Can you work these out from the model? Positions are in its coordinate system, mm. A direction names the side the tool comes from. Coordinates: 2 decimals unless noted, no trailing zeros. Order: outer loops, then holes, each group sorted by start corner. A loop starts at its lowest first (then second) coordinate and runs counter-clockwise, first axis right, second up. Notation, with made-up numbers: (-9.5, 14) -> (-4.5, 14) arc R26 cw to (-4.5, 46) -> close; hole circle Ø5 at (-32.75, 27.5). An arc over 180 degrees is marked (long way). Write item = value, one per line.
```python
from build123d import *

# Parameters (mm, degrees)
F0_W     = 7.62
F0_H     = 12.7
F1_DEPTH = 5.08
F2_W     = 5.08
F2_H     = 2.54
F3_DEPTH = 25.4
F5_DEPTH = 2.54


# Not quite as in the source:
# - a feature names something its author has since deleted; it is built from what else it names


with BuildPart() as f1:
    # F0 (on Top) → F1 (new body)
    with BuildSketch(Plane.XY):
        with Locations((-65.9446567297, 13.238232059)):
            Rectangle(F0_W, F0_H)
    extrude(amount=F1_DEPTH)

    # F2 (on face) → F3 (join)
    with BuildSketch(Plane(origin=(-69.7546567297, 0, 0), x_dir=(0, -1, 0), z_dir=(-1, 0, 0))):
        with Locations((-13.238232059, 1.27)):
            Rectangle(F2_W, F2_H)
    extrude(amount=F3_DEPTH)

    # F4 (on face) → F5 (join)
    with BuildSketch(Plane(origin=(0, 0, 0), x_dir=(1, 0, 0), z_dir=(0, 0, -1))):
        with BuildLine():
            Line((-93.5208049366, -15.778232059), (-95.1546567297, -15.778232059))
            Line((-95.1546567297, -15.778232059), (-95.1546567297, -10.698232059))
            ThreePointArc((-95.1546567297, -10.698232059), (-100.7342725481, -24.1686162406), (-114.2046567297, -29.748232059))
            Line((-114.2046567297, -29.748232059), (-114.2046567297, -31.9967795447))
            ThreePointArc((-114.2046567297, -31.9967795447), (-101.0625202258, -27.4586727786), (-93.5208049366, -15.778232059))
        make_face()
    extrude(amount=-F5_DEPTH)


solid = f1.part
```
Item 1: If we mould it in two halves opening along X, with no side actions, what happens to faces 1 (the flat face through (-66, 6.888, 3)), 2 (the flat face through (-81, 15.778, 1)), 3 (the flat face through (-62.135, 13, 3))? For each: pulls with the +X half, pulls with the -X half, needs draft (parallel to the pull), parting line crosses it, or undercut.
A:
face_1 = needs draft
face_2 = undercut
face_3 = pulls with the +X half
Item 2: I want a section at D-D, the plane z = 3.4. Please give me the cut outline in (x, y), plus the area to 3 significant figures.
A:
outline = (-69.75, 6.89) -> (-62.13, 6.89) -> (-62.13, 19.59) -> (-69.75, 19.59) -> close
area = 96.8 mm2
Item 3: I want a section at B-B, the plane y = 17.25. Please give me the cut outline in (x, z), plus the area to 3 significant figures.
A:
outline = (-96.32, 0) -> (-93.94, 0) -> (-93.94, 2.54) -> (-96.32, 2.54) -> close; (-69.75, 0) -> (-62.13, 0) -> (-62.13, 5.08) -> (-69.75, 5.08) -> close
area = 44.7 mm2
Item 4: I want a section at A-A, the plane z = 0.65. Please give me the cut outline in (x, y), plus the area to 3 significant figures.
A:
outline = (-114.2, 29.75) arc R19.05 cw to (-95.15, 10.7) -> (-69.75, 10.7) -> (-69.75, 6.89) -> (-62.13, 6.89) -> (-62.13, 19.59) -> (-69.75, 19.59) -> (-69.75, 15.78) -> (-93.52, 15.78) arc R21.3 ccw to (-114.2, 32) -> close
area = 287 mm2
Item 5: If I drill on probe 1 along X at (y, z) = (16, 1.85); probe 2 along X at (y, z) = (16.25, 1.7); probe 3 along Y at (x, z) = (-73, 0.6), over which ranges is the centre line in solid material (lowest first)?
A:
probe_1 = -95.91 to -93.58, -69.75 to -62.13
probe_2 = -95.98 to -93.64, -69.75 to -62.13
probe_3 = 10.7 to 15.78
Item 6: I'm going to push flat-ended pins straight in: P1, Ø1.5, axis at x = -66, z = 3, coming from the +Y side; P2, Ø1.3, axis at x = -77, z = 1, coming from the -Y side; P3, Ø1, axis at x = -99.5, z = 2.5, coming from the +Y side; P4, Ø1.5, axis at y = 29, z = 4.5, coming from the -X side. Where does each tip first touch, or does it pass through?
A:
P1 = 19.59
P2 = 10.7
P3 = 26.57
P4 = through
Item 7: I want a section at C-C, the plane x = -86.5. Please give me the cut outline in (y, z).
A:
outline = (10.7, 0) -> (15.78, 0) -> (15.78, 2.54) -> (10.7, 2.54) -> close
Item 8: For faces 4 (the flat face through (-82, 10.698, 1)), 5 (the flat face through (-89, 14, 2.54)), 6 (the flat face through (-69.755, 13, 3)), 7 (the flat face through (-66, 19.588, 3)), which set-ups out of +Z, -Z, +X, -X, +Y, -Y let a thin tool reach every point of the face, with its end or its side?
A:
face_4 = +Z, -Z, -X, -Y
face_5 = +Z, -X, +Y, -Y
face_6 = +Z
face_7 = +Z, -Z, +X, +Y
